from build123d import *

# Parameters (mm, degrees)
EXTRUDE_THIN1_DEPTH            = 80
BOSS_EXTRUDE2_DEPTH            = 20
SKETCH3_R                      = 1.75
SKETCH3_R_2                    = 1.7500092
SKETCH3_R_3                    = 1.25
CUT_EXTRUDE1_DEPTH             = 10
CUT_EXTRUDE2_REACH             = 122
SKETCH6_R                      = 2
BOSS_EXTRUDE3_DEPTH            = 3
FILLET1_R                      = 3
FILLET2_R                      = 3
TAP_DRILL_FOR_M2_5X0_45_TAP1_D = 2.05


with BuildPart() as part:
    # Sketch1 → Extrude-Thin1 (new body)
    with BuildSketch(Plane.XY):
        with BuildLine():
            Line((29, 86), (-81, 86))
            ThreePointArc((-81, 86), (-84.535533906, 84.535533906), (-86, 81))
            Line((-86, 81), (-86, -29))
            ThreePointArc((-86, -29), (-84.535533906, -32.535533906), (-81, -34))
            Line((-81, -34), (29, -34))
            ThreePointArc((29, -34), (32.535533906, -32.535533906), (34, -29))
            Line((34, -29), (34, 81))
            ThreePointArc((34, 81), (32.535533906, 84.535533906), (29, 86))
        make_face()
        with BuildLine():
            Line((29, 83.5), (-81, 83.5))
            ThreePointArc((-81, 83.5), (-82.767766953, 82.767766953), (-83.5, 81))
            Line((-83.5, 81), (-83.5, -29))
            ThreePointArc((-83.5, -29), (-82.767766953, -30.767766953), (-81, -31.5))
            Line((-81, -31.5), (29, -31.5))
            ThreePointArc((29, -31.5), (30.767766953, -30.767766953), (31.5, -29))
            Line((31.5, -29), (31.5, 81))
            ThreePointArc((31.5, 81), (30.767766953, 82.767766953), (29, 83.5))
        make_face(mode=Mode.SUBTRACT)
    extrude(amount=EXTRUDE_THIN1_DEPTH)

    # Sketch2 → Boss-Extrude2 (add)
    with BuildSketch(Plane.XY):
        with BuildLine():
            Line((29, -24), (31.5, -24))
            Line((31.5, -24), (31.5, -29))
            ThreePointArc((31.5, -29), (30.767766953, -30.767766953), (29, -31.5))
            Line((29, -31.5), (24, -31.5))
            Line((24, -31.5), (24, -29))
            ThreePointArc((24, -29), (25.464466094, -25.464466094), (29, -24))
        make_face()
        with BuildLine():
            Line((-76, -29), (-76, -31.5))
            Line((-76, -31.5), (-81, -31.5))
            ThreePointArc((-81, -31.5), (-82.767766953, -30.767766953), (-83.5, -29))
            Line((-83.5, -29), (-83.5, -24))
            Line((-83.5, -24), (-81, -24))
            ThreePointArc((-81, -24), (-77.464466094, -25.464466094), (-76, -29))
        make_face()
        with BuildLine():
            Line((-81, 76), (-83.5, 76))
            Line((-83.5, 76), (-83.5, 81))
            ThreePointArc((-83.5, 81), (-82.767766953, 82.767766953), (-81, 83.5))
            Line((-81, 83.5), (-76, 83.5))
            Line((-76, 83.5), (-76, 81))
            ThreePointArc((-76, 81), (-77.464466094, 77.464466094), (-81, 76))
        make_face()
        with BuildLine():
            Line((24, 81), (24, 83.5))
            Line((24, 83.5), (29, 83.5))
            ThreePointArc((29, 83.5), (30.767766953, 82.767766953), (31.5, 81))
            Line((31.5, 81), (31.5, 76))
            Line((31.5, 76), (29, 76))
            ThreePointArc((29, 76), (25.464466094, 77.464466094), (24, 81))
        make_face()
    extrude(amount=BOSS_EXTRUDE2_DEPTH)

    # Sketch3 → Cut-Extrude1 (cut)
    with BuildSketch(Plane.XZ.offset(34)):
        with Locations((9.866177282, 61.657658655)):
            Circle(SKETCH3_R)
        with Locations((8.690958198, 13.395257553)):
            Circle(SKETCH3_R)
        with Locations((-42.193745622, 56.475407474)):
            Circle(SKETCH3_R_2)
        with Locations((-42.138873878, 28.535461355)):
            Circle(SKETCH3_R_2)
        with Locations((-65.153703669, 54.105224901)):
            Circle(SKETCH3_R_3)
        with Locations((-65.153703669, 20.105224901)):
            Circle(SKETCH3_R_3)
    extrude(amount=-CUT_EXTRUDE1_DEPTH, mode=Mode.SUBTRACT)

    # Sketch4 → Cut-Extrude2 (cut, up to next)
    with BuildSketch(Plane.XZ.offset(34), mode=Mode.PRIVATE) as cut_extrude2_sk1:
        with BuildLine():
            Line((-6, 0), (-46, 0))
            Line((-46, 0), (-46, 7))
            ThreePointArc((-46, 7), (-45.121320344, 9.121320344), (-43, 10))
            Line((-43, 10), (-9, 10))
            ThreePointArc((-9, 10), (-6.878679656, 9.121320344), (-6, 7))
            Line((-6, 7), (-6, 0))
        make_face()
    cut_extrude2_tool1 = extrude(cut_extrude2_sk1.sketch, amount=-CUT_EXTRUDE2_REACH, mode=Mode.PRIVATE) & part.part
    add(cut_extrude2_tool1.solids().sort_by_distance((-26, -34, 4.957778))[0], mode=Mode.SUBTRACT)

    # Sketch6 → Boss-Extrude3 (add)
    with BuildSketch(Plane.XY.offset(80)):
        with BuildLine():
            Line((-86, -14), (-86, 1))
            Line((-86, 1), (-95, 1))
            ThreePointArc((-95, 1), (-97.121320344, 0.121320344), (-98, -2))
            Line((-98, -2), (-98, -11))
            ThreePointArc((-98, -11), (-97.121320344, -13.121320344), (-95, -14))
            Line((-95, -14), (-86, -14))
        make_face()
        with Locations((-93, -6.5)):
            Circle(SKETCH6_R, mode=Mode.SUBTRACT)
        with BuildLine():
            Line((43, 1), (34, 1))
            Line((34, 1), (34, -14))
            Line((34, -14), (43, -14))
            ThreePointArc((43, -14), (45.121320344, -13.121320344), (46, -11))
            Line((46, -11), (46, -2))
            ThreePointArc((46, -2), (45.121320344, 0.121320344), (43, 1))
        make_face()
        with Locations((41, -6.5)):
            Circle(SKETCH6_R, mode=Mode.SUBTRACT)
        with BuildLine():
            Line((46, 54), (46, 63))
            ThreePointArc((46, 63), (45.121320344, 65.121320344), (43, 66))
            Line((43, 66), (34, 66))
            Line((34, 66), (34, 51))
            Line((34, 51), (43, 51))
            ThreePointArc((43, 51), (45.121320344, 51.878679656), (46, 54))
        make_face()
        with Locations((41, 58.5)):
            Circle(SKETCH6_R, mode=Mode.SUBTRACT)
        with BuildLine():
            Line((-86, 51), (-86, 66))
            Line((-86, 66), (-95, 66))
            ThreePointArc((-95, 66), (-97.121320344, 65.121320344), (-98, 63))
            Line((-98, 63), (-98, 54))
            ThreePointArc((-98, 54), (-97.121320344, 51.878679656), (-95, 51))
            Line((-95, 51), (-86, 51))
        make_face()
        with Locations((-93, 58.5)):
            Circle(SKETCH6_R, mode=Mode.SUBTRACT)
    extrude(amount=-BOSS_EXTRUDE3_DEPTH)

    # Fillet1
    fillet1_edges = [part.edges().sort_by_distance(p)[0] for p in [
        (-86, 1, 78.5),
        (-86, -14, 78.5),
        (34, -14, 78.5),
        (34, 1, 78.5),
        (34, 51, 78.5),
        (34, 66, 78.5),
        (-86, 66, 78.5),
        (-86, 51, 78.5),
    ]]
    fillet(fillet1_edges, radius=FILLET1_R)

    # Fillet2
    fillet2_edges = [part.edges().sort_by_distance(p)[0] for p in [
        (34, 58.5, 77),
        (34, -6.5, 77),
        (-86, 58.5, 77),
        (-86, -6.5, 77),
    ]]
    fillet(fillet2_edges, radius=FILLET2_R)

    # Tap Drill for M2.5x0.45 Tap1 (through all)
    with Locations(Plane(origin=(0, 0, 0), x_dir=(-1, 0, 0), z_dir=(0, 0, -1))):
        with Locations((81, -29), (81, 81), (-29, -29), (-29, 81)):
            Hole(TAP_DRILL_FOR_M2_5X0_45_TAP1_D / 2)


solid = part.part
Work out the finished part from the listing and answer in its coordinate system (mm). A direction names the side the tool comes from. Round coordinates to 2 decimals unless told otherwise and drop trailing zeros. Order: outer loops, then holes, each group sorted by start corner. A loop starts at its lowest first (then second) coordinate and runs counter-clockwise, first axis right, second up. Notation, with made-up numbers: M 59.5,14 L 77.5,14 A24 cw 77.5,32 Z; hole C -25.75,25 d4. An arc over 180 degrees is marked long. One line per item, written item: value.
Q1. Find section D-D on z = 65.5. Write down the section's boundary in (x, y).
Derived:
outline: M -86,-29 A5 ccw -81,-34 L 29,-34 A5 ccw 34,-29 L 34,81 A5 ccw 29,86 L -81,86 A5 ccw -86,81 Z; hole M -83.5,-29 A2.5 ccw -81,-31.5 L 29,-31.5 A2.5 ccw 31.5,-29 L 31.5,81 A2.5 ccw 29,83.5 L -81,83.5 A2.5 ccw -83.5,81 Z
Q2. Find section B-B on y = -6.5. Write down the section's boundary in (x, z).
Derived:
outline: M -98,77 L -95,77 L -95,80 L -98,80 Z; M -91,77 L -89,77 A3 cw -86,74 L -86,0 L -83.5,0 L -83.5,80 L -91,80 Z; M 31.5,0 L 34,0 L 34,74 A3 cw 37,77 L 39,77 L 39,80 L 31.5,80 Z; M 43,77 L 46,77 L 46,80 L 43,80 Z
Q3. Determine the mould class of faces 6 (the face through (-42.42, -32.77, 58.21)), 7 (the face through (32, -33, 39)), 8 (the face through (25, -26, 10)), 9 (the face through (-84, 85, 39)) for opening direction Y: released by +Y, released by -Y, zero draft, split by the parting line, or undercut.
Derived:
face 6: zero draft
face 7: released by -Y
face 8: undercut
face 9: released by +Y
Q4. For faces 1 (the face through (10.674, -32.768, 60.105)), 2 (the face through (42.4, -4.7, 77)), 3 (the face through (-95, 60, 77)), 4 (the face through (28, -28, 20)), 5 (the face through (-78, -25, 10)), determine the directions among +Z, -Z, +X, -X, +Y, -Y from which every point of the face is accessible in a straight line to the end or side of a thin tool.
Derived:
face 1: -Y
face 2: -Z, +X, +Y, -Y
face 3: -Z, -X, +Y, -Y
face 4: +Z
face 5: +Z, -Z
Q5. Straight lines are drawn through the part: line 1 (Y direction, x = 41, z = 78); line 2 (X direction, y = 17, z = 37.5); line 3 (Y direction, x = -35, z = 30.5). For each, find the intervals that lie inside material, in ascending order.
Derived:
line 1: -14 to -8.5, -4.5 to 1, 51 to 56.5, 60.5 to 66
line 2: -86 to -83.5, 31.5 to 34
line 3: -34 to -31.5, 83.5 to 86
Q6. Flat-ended cylindrical pins translate along their axes: pin 1 (1.2 mm diameter, centred on y = 82, z = 7, fed in from -X); pin 2 (3 mm diameter, centred on x = 9.87, z = 61.66, fed in from -Y); pin 3 (3 mm diameter, centred on x = 31, z = 12.5, fed in from +Y). Find the tip coordinate at first contact, or state that the pin passes through.
Derived:
pin 1: x = -85.98
pin 2: y = 83.5
pin 3: y = 85.97
Q7. Find section C-C on x = -93. Write down the section's boundary in (y, z), then the cut area to 3 significant figures.
Derived:
outline: M -14,77 L -8.5,77 L -8.5,80 L -14,80 Z; M -4.5,77 L 1,77 L 1,80 L -4.5,80 Z; M 51,77 L 56.5,77 L 56.5,80 L 51,80 Z; M 60.5,77 L 66,77 L 66,80 L 60.5,80 Z
area: 66.0 mm²
Q8. Find section A-A on x = -70. Write down the section's boundary in (y, z), then the cut area to 3 significant figures.
Derived:
outline: M -34,0 L -31.5,0 L -31.5,80 L -34,80 Z; M 83.5,0 L 86,0 L 86,80 L 83.5,80 Z
area: 400 mm²
